Read the model definition and answer for the solid it produces. Units are mm, in the model's axes. Give positions to 0.01 mm unless a question says otherwise; leave off trailing zeros. Loops run counter-clockwise (first coordinate to the right, second up) from the corner with the lowest first, then second, coordinate; pieces in that order, holes last. Notation, with made-up numbers: (-13.5, -35.75) -> (5.5, -35.75) arc R23 ccw to (5.5, -0.75) -> close; hole circle Ø7 at (77, 57.5). An arc over 180 degrees is marked (long way). One line per item, written item: value. Start each with the question number.
from build123d import *

# Parameters (mm, degrees)
SKETCH_W          = 130
SKETCH_H          = 107
PAD_DEPTH         = 1
SKETCH001_W       = 130
SKETCH001_H       = 1
PAD001_DEPTH      = 2
SKETCH002_W       = 130
SKETCH002_H       = 1
PAD002_DEPTH      = 2
SKETCH003_W       = 130
SKETCH003_H       = 1
PAD003_DEPTH      = 2
SKETCH004_W       = 130
SKETCH004_H       = 1
PAD004_DEPTH      = 2
SKETCH005_W       = 90
SKETCH005_H       = 65
POCKET_DEPTH      = 1.001
POCKET_DEPTH_BACK = 2.001


with BuildPart() as part:
    # Sketch → Pad (new body)
    with BuildSketch(Plane.XY):
        with Locations((65, 53.5)):
            Rectangle(SKETCH_W, SKETCH_H)
    extrude(amount=-PAD_DEPTH)

    # Sketch001 → Pad001 (join)
    with BuildSketch(Plane.XY):
        with Locations((65, 106.5)):
            Rectangle(SKETCH001_W, SKETCH001_H)
    extrude(amount=PAD001_DEPTH)

    # Sketch002 → Pad002 (join)
    with BuildSketch(Plane.XY):
        with Locations((65, 104)):
            Rectangle(SKETCH002_W, SKETCH002_H)
    extrude(amount=PAD002_DEPTH)

    # Sketch003 → Pad003 (join)
    with BuildSketch(Plane.XY):
        with Locations((65, 3)):
            Rectangle(SKETCH003_W, SKETCH003_H)
    extrude(amount=PAD003_DEPTH)

    # Sketch004 → Pad004 (join)
    with BuildSketch(Plane.XY):
        with Locations((65, 0.5)):
            Rectangle(SKETCH004_W, SKETCH004_H)
    extrude(amount=PAD004_DEPTH)

    # Sketch005 → Pocket (cut, two sides)
    with BuildSketch(Plane.XY) as pocket_sk:
        with Locations((65, 53.5)):
            Rectangle(SKETCH005_W, SKETCH005_H)
    extrude(amount=-POCKET_DEPTH, mode=Mode.SUBTRACT)
    extrude(pocket_sk.sketch, amount=POCKET_DEPTH_BACK, mode=Mode.SUBTRACT)


solid = part.part
Item 1: Section A-A, the plane z = 0.95 is taken. Determine the outline of the cut face in (x, y).
Item 2: A flat-ended cylindrical pin translates along its axis: pin 1 (0.8 mm diameter, centred on x = 80.5, y = 2, fed in from +Z). Find the tip coordinate at first contact, or state that the pin passes through.
Item 3: Section D-D, the plane x = 11 is taken. Determine the outline of the cut face in (y, z).
Item 4: Determine the mould class of faces 1 (the flat face through (64, 107, 0)), 2 (the flat face through (0, 53.3, -0.6)), 3 (the flat face through (64, 0, 0)), 4 (the flat face through (64, 88, 0)) for opening direction Y: pulls with the +Y half, pulls with the -Y half, needs draft (parallel to the pull), parting line crosses it, or undercut.
Item 5: Section C-C, the plane x = 38 is taken. Determine the outline of the cut face in (y, z).
Item 6: Section B-B, the plane y = 68.5 is taken. Determine the outline of the cut face in (x, z).
Item 7: Consider L1, parallel to Y at x = 25, z = 0.05; L2, parallel to X at y = 79.5, z = -0.5; L3, parallel to Y at x = 57, z = -0.4. Determine where each line is inside the solid, lowest interval first. Write a range as [from, to].
Computed values:
1. outline: (0, 0) -> (130, 0) -> (130, 1) -> (0, 1) -> close; (0, 2.5) -> (130, 2.5) -> (130, 3.5) -> (0, 3.5) -> close; (0, 103.5) -> (130, 103.5) -> (130, 104.5) -> (0, 104.5) -> close; (0, 106) -> (130, 106) -> (130, 107) -> (0, 107) -> close
2. pin 1: z = 0
3. outline: (0, -1) -> (107, -1) -> (107, 2) -> (106, 2) -> (106, 0) -> (104.5, 0) -> (104.5, 2) -> (103.5, 2) -> (103.5, 0) -> (3.5, 0) -> (3.5, 2) -> (2.5, 2) -> (2.5, 0) -> (1, 0) -> (1, 2) -> (0, 2) -> close
4. face 1: pulls with the +Y half
4. face 2: needs draft
4. face 3: pulls with the -Y half
4. face 4: undercut
5. outline: (0, -1) -> (21, -1) -> (21, 0) -> (3.5, 0) -> (3.5, 2) -> (2.5, 2) -> (2.5, 0) -> (1, 0) -> (1, 2) -> (0, 2) -> close; (86, -1) -> (107, -1) -> (107, 2) -> (106, 2) -> (106, 0) -> (104.5, 0) -> (104.5, 2) -> (103.5, 2) -> (103.5, 0) -> (86, 0) -> close
6. outline: (0, -1) -> (20, -1) -> (20, 0) -> (0, 0) -> close; (110, -1) -> (130, -1) -> (130, 0) -> (110, 0) -> close
7. L1: [0, 1], [2.5, 3.5], [103.5, 104.5], [106, 107]
7. L2: [0, 20], [110, 130]
7. L3: [0, 21], [86, 107]
